Verification items for the finished model (mm, model axes). A direction names the side the tool comes from. Coordinates: 2 decimals unless noted, no trailing zeros. Write each loop counter-clockwise with the first axis right and the second up, starting at its lowest first coordinate (ties: lowest second). Pieces come first, ordered by that corner, then holes. Notation, with made-up numbers: (18, 26.5) -> (64, 26.5) arc R23 ccw to (64, 47.5) -> close; hole circle Ø8 at (36.5, -16). An arc over 180 degrees is marked (long way). Use a Markdown table: item, result. Add a question column.
from build123d import *

# Parameters (mm, degrees)
BOSS_EXTRUDE1_DEPTH = 2


with BuildPart() as part:
    # Sketch1 → Boss-Extrude1 (new body)
    with BuildSketch(Plane.XY):
        with BuildLine():
            Line((13.368173221, 13.377065301), (4.368173221, 13.377065301))
            Line((4.368173221, 13.377065301), (4.368173221, 5.377065301))
            Line((4.368173221, 5.377065301), (6.368173221, 5.377065301))
            ThreePointArc((6.368173221, 5.377065301), (6.80751305, 6.437725473), (7.868173221, 6.877065301))
            Line((7.868173221, 6.877065301), (9.368173221, 6.877065301))
            Line((9.368173221, 6.877065301), (9.368173221, 9.877956548))
            ThreePointArc((9.368173221, 9.877956548), (8.59232295, 10.627510924), (9.368173221, 11.377065301))
            Line((9.368173221, 11.377065301), (9.868173221, 11.377065301))
            ThreePointArc((9.868173221, 11.377065301), (10.618173221, 12.127065301), (11.368173221, 11.377065301))
            Line((11.368173221, 11.377065301), (11.368173221, 10.877065301))
            Line((11.368173221, 10.877065301), (13.368173221, 11.377065301))
            Line((13.368173221, 11.377065301), (13.368173221, 13.377065301))
        make_face()
    boss_extrude1 = extrude(amount=BOSS_EXTRUDE1_DEPTH)

    # Mirror1: Boss-Extrude1 across plane
    add(boss_extrude1.mirror(Plane(origin=(6.368173221, 5.377065301, 2), x_dir=(0, 0, 1), z_dir=(0, 1, 0))))


solid = part.part
1) Gauge pin test, flat end, axial feed: pin 1 (0.6 mm diameter, centred on y = 2, z = 1, fed in from +X). Record the tip position at first contact, or that the pin passes through.
2) Thickness scan on L1, parallel to Y at x = 9.5, z = 1.45; L2, parallel to Y at x = 8.75, z = 0.8; L3, parallel to Y at x = 9, z = 0.7. Record the ranges inside material, lowest first.
3) Cross-section at D-D on y = 2.75. Record the boundary of the cut face in (x, z), then the cut area to 3 significant figures.
4) Cross-section at A-A on x = 8.25. Record the boundary of the cut face in (y, z).
5) Set-up check for faces 4 (the face through (12.354, 11.124, 0.986)), 5 (the face through (8.593, 10.611, 0.986)), 6 (the face through (4.368, 5, 1)): record each of +Z, -Z, +X, -X, +Y, -Y from which the full face is reachable in a straight line by a thin tool's end or side.
6) Cross-section at B-B on z = 0.25. Record the boundary of the cut face in (x, y), then the cut area to 3 significant figures.
7) Release check for a two-part mould opening along Y. For faces 1 (the face through (10.602, 12.127, 0.986)), 2 (the face through (9, -2.623, 1)), 3 (the face through (6, 5, 0)) record: released by +Y, released by -Y, zero draft, split by the parting line, or undercut.
8) Cross-section at C-C on x = 13. Record the boundary of the cut face in (y, z).
Returned:
| question | item | result |
|---|---|---|
| 1 | pin 1 | stops at x = 9.37 |
| 2 | L1 | y = -2.62 to -0.62, 11.38 to 13.38 |
| 2 | L2 | y = -2.62 to -0.33, 0.59 to 3.88, 6.88 to 10.17, 11.09 to 13.38 |
| 2 | L3 | y = -2.62 to -0.54, 0.79 to 3.88, 6.88 to 9.96, 11.29 to 13.38 |
| 3 | outline | (4.37, 0) -> (9.37, 0) -> (9.37, 2) -> (4.37, 2) -> close |
| 3 | area | 10.0 mm² |
| 4 | outline | (-2.62, 0) -> (3.88, 0) -> (3.88, 2) -> (-2.62, 2) -> close; (6.88, 0) -> (13.38, 0) -> (13.38, 2) -> (6.88, 2) -> close |
| 5 | face 4 | +Z, -Z, +X |
| 5 | face 5 | +Z, -Z |
| 5 | face 6 | +Z, -Z, -X, +Y, -Y |
| 6 | outline | (4.37, -2.62) -> (13.37, -2.62) -> (13.37, -0.62) -> (11.37, -0.12) -> (11.37, -0.62) arc R0.75 cw to (9.87, -0.62) -> (9.37, -0.62) arc R0.75 cw (long way) to (9.37, 0.88) -> (9.37, 3.88) -> (7.87, 3.88) arc R1.5 cw to (7.87, 6.88) -> (9.37, 6.88) -> (9.37, 9.88) arc R0.75 cw (long way) to (9.37, 11.38) -> (9.87, 11.38) arc R0.75 cw to (11.37, 11.38) -> (11.37, 10.88) -> (13.37, 11.38) -> (13.37, 13.38) -> (4.37, 13.38) -> close |
| 6 | area | 85.4 mm² |
| 7 | face 1 | undercut |
| 7 | face 2 | released by -Y |
| 7 | face 3 | zero draft |
| 8 | outline | (-2.62, 0) -> (-0.53, 0) -> (-0.53, 2) -> (-2.62, 2) -> close; (11.29, 0) -> (13.38, 0) -> (13.38, 2) -> (11.29, 2) -> close |
